For this review, take the finished solid that the model builds, in its own axes (mm). Round coordinates to 2 decimals unless told otherwise and drop trailing zeros. Use one line per item in the form item = value. Start each with the question number.
Item 1: Add section A-A (z = 0.1). Count the separate pieces of the cut face and the enclosed holes in it, and give its area (3 significant figures).
Item 2: For line 1 (Y direction, x = -1, z = 0.1); line 2 (X direction, y = 7, z = 0.2); line 3 (Y direction, x = -2.5, z = 0.15), list the stretches that pass through material, from the lowest coordinate up. Write a range as [from, to].
Item 3: For P1, Ø6, axis at x = -18.5, y = 7, coming from the -Z side; P2, Ø12, axis at x = 7, y = 4.5, coming from the +Z side, all flat-tipped, find the tip position at first contact; note any pin that passes through.
from build123d import *

# Parameters (mm, degrees)
SKETCH4_R           = 28.575
BOSS_EXTRUDE2_DEPTH = 0.254
SKETCH5_R           = 15.875
CUT_EXTRUDE5_DEPTH  = 1.254
CUT_EXTRUDE6_DEPTH  = 1.254
CUT_EXTRUDE11_DEPTH = 1.254


with BuildPart() as part:
    # Sketch4 → Boss-Extrude2 (new body)
    with BuildSketch(Plane.XY):
        Circle(SKETCH4_R)
    extrude(amount=BOSS_EXTRUDE2_DEPTH)

    # Sketch5 → Cut-Extrude5 (cut, through all)
    with BuildSketch(Plane.XY.offset(0.254)):
        Circle(SKETCH5_R)
    extrude(amount=-CUT_EXTRUDE5_DEPTH, mode=Mode.SUBTRACT)

    # Sketch6 → Cut-Extrude6 (cut, through all)
    with BuildSketch(Plane.XY.offset(0.254)):
        with BuildLine():
            ThreePointArc((19.038143, 19.038142953), (12.392753451, 19.038142981), (12.392753462, 12.392753432))
            ThreePointArc((12.392753462, 12.392753432), (16.1919128, 6.706909562), (17.526, -5.71e-07))
            ThreePointArc((17.526, -5.71e-07), (22.224999847, -4.699), (26.924, -8.77e-07))
            ThreePointArc((26.924, -8.77e-07), (24.874532708, 10.303368312), (19.038143, 19.038142953))
        make_face()
        with BuildLine():
            ThreePointArc((19.038142953, -19.038143), (19.038142981, -12.392753451), (12.392753432, -12.392753462))
            ThreePointArc((12.392753432, -12.392753462), (6.706909562, -16.1919128), (-5.71e-07, -17.526))
            ThreePointArc((-5.71e-07, -17.526), (-4.699, -22.224999847), (-8.77e-07, -26.924))
            ThreePointArc((-8.77e-07, -26.924), (10.303368312, -24.874532708), (19.038142953, -19.038143))
        make_face()
        with BuildLine():
            ThreePointArc((-19.038143, -19.038142953), (-12.392753451, -19.038142981), (-12.392753462, -12.392753432))
            ThreePointArc((-12.392753462, -12.392753432), (-16.1919128, -6.706909562), (-17.526, 5.71e-07))
            ThreePointArc((-17.526, 5.71e-07), (-22.224999847, 4.699), (-26.924, 8.77e-07))
            ThreePointArc((-26.924, 8.77e-07), (-24.874532708, -10.303368312), (-19.038143, -19.038142953))
        make_face()
        with BuildLine():
            ThreePointArc((-19.038142953, 19.038143), (-19.038142981, 12.392753451), (-12.392753432, 12.392753462))
            ThreePointArc((-12.392753432, 12.392753462), (-6.706909562, 16.1919128), (5.71e-07, 17.526))
            ThreePointArc((5.71e-07, 17.526), (4.699, 22.224999847), (8.77e-07, 26.924))
            ThreePointArc((8.77e-07, 26.924), (-10.303368312, 24.874532708), (-19.038142953, 19.038143))
        make_face()
    extrude(amount=-CUT_EXTRUDE6_DEPTH, mode=Mode.SUBTRACT)

    # Sketch8 → Cut-Extrude11 (cut, through all)
    with BuildSketch(Plane.XY.offset(0.254)):
        Polygon((27.472529104, 10.004856053), (26.500513186, 12.351510066), (25.327186179, 11.865502107), (26.299202097, 9.518848094), align=None)
        Polygon((-10.004856053, 27.472529104), (-12.351510066, 26.500513186), (-11.865502107, 25.327186179), (-9.518848094, 26.299202097), align=None)
        Polygon((-26.500513186, 12.351510066), (-27.472529104, 10.004856053), (-26.299202097, 9.518848094), (-25.327186179, 11.865502107), align=None)
        Polygon((-27.472529104, -10.004856053), (-26.500513186, -12.351510066), (-25.327186179, -11.865502107), (-26.299202097, -9.518848094), align=None)
        Polygon((-12.351510066, -26.500513186), (-10.004856053, -27.472529104), (-9.518848094, -26.299202097), (-11.865502107, -25.327186179), align=None)
        Polygon((10.004856053, -27.472529104), (12.351510066, -26.500513186), (11.865502107, -25.327186179), (9.518848094, -26.299202097), align=None)
        Polygon((26.500513186, -12.351510066), (27.472529104, -10.004856053), (26.299202097, -9.518848094), (25.327186179, -11.865502107), align=None)
        Polygon((12.351510066, 26.500513186), (10.004856053, 27.472529104), (9.518848094, 26.299202097), (11.865502107, 25.327186179), align=None)
    extrude(amount=-CUT_EXTRUDE11_DEPTH, mode=Mode.SUBTRACT)


solid = part.part
Calculated:
q1.separate_pieces = 1
q1.enclosed_holes = 5
q1.area = 827 mm^2
q2.line_1 = [-28.56, -26.82], [-17.63, -15.84], [15.84, 17.5], [26.91, 28.56]
q2.line_2 = [-27.7, -14.25], [14.25, 16.07], [26, 27.7]
q2.line_3 = [-28.47, -26.2], [-18.25, -15.68], [15.68, 17.35], [26.81, 28.47]
q3.P1 = 0
q3.P2 = through
